Check sheet for the modelled part. Datum: model origin and axes. Units: mm. A direction names the side the tool comes from. Round coordinates to 2 decimals unless told otherwise and drop trailing zeros. One line per item, written item: value. Start each with the question number.
(1) Access from +Z, -Z, +X, -X, +Y, -Y to the whole of each face (thin tool, end or side, straight path). Record for faces 4 (the face through (-1, 2, -85)), 5 (the face through (46, 2, 38)).
(2) Thickness scan on L1, parallel to X at y = 2.9, z = 40; L2, parallel to X at y = 1.05, z = -40; L3, parallel to Z at x = 45.5, y = 2.6. Record the ranges inside material, lowest first.
(3) Release check for a two-part mould opening along X. For faces 1 (the face through (-45.189, 3.014, 42.575)), 2 (the face through (85, 2, 1)), 3 (the face through (-1, 0, -1)) record: released by +X, released by -X, zero draft, split by the parting line, or undercut.
(4) Depth check by flat-ended pin: pin 1 Ø2.5 at (x, z) = (-46.5, 41) entering from +Y. Enter the tip coordinate at first touch or a pass-through.
from build123d import *

# Parameters (mm, degrees)
SKETCH1_W           = 170
SKETCH1_H           = 170
BOSS_EXTRUDE1_DEPTH = 4
CUT_EXTRUDE1_REACH  = 122.275
SKETCH2_R           = 1.6
SKETCH2_3_R         = 2.7
SKETCH2_3_R_2       = 1.6
CUT_EXTRUDE2_DEPTH  = 2


with BuildPart() as part:
    # Sketch1 → Boss-Extrude1 (new body)
    with BuildSketch(Plane(origin=(0, 0, 0), x_dir=(1, 0, 0), z_dir=(0, 1, 0))):
        Rectangle(SKETCH1_W, SKETCH1_H)
    extrude(amount=BOSS_EXTRUDE1_DEPTH)

    # Sketch2 → Cut-Extrude1 (cut, up to next)
    with BuildSketch(Plane(origin=(0, 4, 0), x_dir=(1, 0, 0), z_dir=(0, 1, 0)), mode=Mode.PRIVATE) as cut_extrude1_sk1:
        with Locations(Location((-46, -40, 0), (0, 0, 270))):
            Circle(SKETCH2_R)
    cut_extrude1_tool1 = extrude(cut_extrude1_sk1.sketch, amount=-CUT_EXTRUDE1_REACH, mode=Mode.PRIVATE) & part.part
    # Sketch2 → Cut-Extrude1 (cut, up to next)
    with BuildSketch(Plane(origin=(0, 4, 0), x_dir=(1, 0, 0), z_dir=(0, 1, 0)), mode=Mode.PRIVATE) as cut_extrude1_sk2:
        with Locations(Location((-46, 40, 0), (0, 0, 270))):
            Circle(SKETCH2_R)
    cut_extrude1_tool2 = extrude(cut_extrude1_sk2.sketch, amount=-CUT_EXTRUDE1_REACH, mode=Mode.PRIVATE) & part.part
    # Sketch2 → Cut-Extrude1 (cut, up to next)
    with BuildSketch(Plane(origin=(0, 4, 0), x_dir=(1, 0, 0), z_dir=(0, 1, 0)), mode=Mode.PRIVATE) as cut_extrude1_sk3:
        with Locations(Location((46, -40, 0), (0, 0, 270))):
            Circle(SKETCH2_R)
    cut_extrude1_tool3 = extrude(cut_extrude1_sk3.sketch, amount=-CUT_EXTRUDE1_REACH, mode=Mode.PRIVATE) & part.part
    # Sketch2 → Cut-Extrude1 (cut, up to next)
    with BuildSketch(Plane(origin=(0, 4, 0), x_dir=(1, 0, 0), z_dir=(0, 1, 0)), mode=Mode.PRIVATE) as cut_extrude1_sk4:
        with Locations(Location((46, 40, 0), (0, 0, 270))):
            Circle(SKETCH2_R)
    cut_extrude1_tool4 = extrude(cut_extrude1_sk4.sketch, amount=-CUT_EXTRUDE1_REACH, mode=Mode.PRIVATE) & part.part
    add(cut_extrude1_tool1.solids().sort_by_distance((-46, 4, 40))[0], mode=Mode.SUBTRACT)
    add(cut_extrude1_tool2.solids().sort_by_distance((-46, 4, -40))[0], mode=Mode.SUBTRACT)
    add(cut_extrude1_tool3.solids().sort_by_distance((46, 4, 40))[0], mode=Mode.SUBTRACT)
    add(cut_extrude1_tool4.solids().sort_by_distance((46, 4, -40))[0], mode=Mode.SUBTRACT)

    # Sketch2_3 → Cut-Extrude2 (cut)
    # profile 1 of 4: a face of its own
    with BuildSketch(Plane(origin=(0, 4, 0), x_dir=(1, 0, 0), z_dir=(0, 1, 0))):
        with Locations(Location((46, 40, 0), (0, 0, 270))):
            Circle(SKETCH2_3_R)
        with Locations(Location((46, 40, 0), (0, 0, 270))):
            Circle(SKETCH2_3_R_2, mode=Mode.SUBTRACT)
    # profile 2 of 4: a face of its own
    with BuildSketch(Plane(origin=(0, 4, 0), x_dir=(1, 0, 0), z_dir=(0, 1, 0))):
        with Locations(Location((-46, 40, 0), (0, 0, 90))):
            Circle(SKETCH2_3_R)
        with Locations(Location((-46, 40, 0), (0, 0, 90))):
            Circle(SKETCH2_3_R_2, mode=Mode.SUBTRACT)
    # profile 3 of 4: a face of its own
    with BuildSketch(Plane(origin=(0, 4, 0), x_dir=(1, 0, 0), z_dir=(0, 1, 0))):
        with Locations(Location((46, -40, 0), (0, 0, 90))):
            Circle(SKETCH2_3_R)
        with Locations(Location((46, -40, 0), (0, 0, 90))):
            Circle(SKETCH2_3_R_2, mode=Mode.SUBTRACT)
    # profile 4 of 4: a face of its own
    with BuildSketch(Plane(origin=(0, 4, 0), x_dir=(1, 0, 0), z_dir=(0, 1, 0))):
        with Locations(Location((-46, -40, 0), (0, 0, 270))):
            Circle(SKETCH2_3_R)
        with Locations(Location((-46, -40, 0), (0, 0, 270))):
            Circle(SKETCH2_3_R_2, mode=Mode.SUBTRACT)
    extrude(amount=-CUT_EXTRUDE2_DEPTH, mode=Mode.SUBTRACT)


solid = part.part
Values found:
1. face 4: -Z, +X, -X, +Y, -Y
1. face 5: +Y
2. L1: -85 to -48.7, -43.3 to 43.3, 48.7 to 85
2. L2: -85 to -47.6, -44.4 to 44.4, 47.6 to 85
2. L3: -85 to -42.65, -37.35 to 37.35, 42.65 to 85
3. face 1: undercut
3. face 2: released by +X
3. face 3: zero draft
4. pin 1: y = 2
